from build123d import *

# Parameters (mm, degrees)
SKETCH_W        = 67.5
SKETCH_H        = 43.5
SKETCH_R        = 2
SKETCH_R_2      = 1.6
SKETCH_W_2      = 7.2
SKETCH_H_2      = 3.2
SKETCH_W_3      = 3.2
SKETCH_H_3      = 7.2
PAD_DEPTH       = 7
PAD001_DEPTH    = 5
SKETCH002_W     = 12
SKETCH002_H     = 12
PAD002_DEPTH    = 12
SKETCH003_R     = 4.2
POCKET_DEPTH    = 5
SKETCH004_R     = 1.7
POCKET001_DEPTH = 5
SKETCH005_R     = 1.7
POCKET002_DEPTH = 5


with BuildPart() as part:
    # Sketch → Pad (new body)
    with BuildSketch(Plane.XY):
        Rectangle(SKETCH_W, SKETCH_H)
        with Locations((0, -4.25)):
            Circle(SKETCH_R, mode=Mode.SUBTRACT)
        with Locations((-15.5, 11.25)):
            Circle(SKETCH_R_2, mode=Mode.SUBTRACT)
        with Locations((15.5, -19.75)):
            Circle(SKETCH_R_2, mode=Mode.SUBTRACT)
        with Locations((15.15, 18.15)):
            Rectangle(SKETCH_W_2, SKETCH_H_2, mode=Mode.SUBTRACT)
        with Locations((-25.15, 18.15)):
            Rectangle(SKETCH_W_2, SKETCH_H_2, mode=Mode.SUBTRACT)
        with Locations((30.15, 5.15)):
            Rectangle(SKETCH_W_3, SKETCH_H_3, mode=Mode.SUBTRACT)
        with Locations((30.15, -13.15)):
            Rectangle(SKETCH_W_3, SKETCH_H_3, mode=Mode.SUBTRACT)
    extrude(amount=PAD_DEPTH)

    # Sketch001 → Pad001 (new body)
    with BuildSketch(Plane.XY.offset(7)):
        Polygon((28.75, -21.75), (33.75, -21.75), (33.75, 21.75), (-33.75, 21.75), (-33.75, -21.75), (-21.75, -21.75), (-21.75, 16.75), (28.75, 16.75), align=None)
    extrude(amount=PAD001_DEPTH)

    # Sketch002 → Pad002 (new body)
    with BuildSketch(Plane.XY.offset(12)):
        with Locations((-27.75, -2)):
            Rectangle(SKETCH002_W, SKETCH002_H)
    extrude(amount=PAD002_DEPTH)

    # Sketch003 → Pocket (cut)
    with BuildSketch(Plane(origin=(-33.75, 0, 0), x_dir=(0, -1, 0), z_dir=(-1, 0, 0))):
        with Locations((2, 18)):
            Circle(SKETCH003_R)
    extrude(amount=-POCKET_DEPTH, mode=Mode.SUBTRACT)

    # Sketch004 → Pocket001 (cut)
    with BuildSketch(Plane(origin=(0, 21.75, 0), x_dir=(-1, 0, 0), z_dir=(0, 1, 0))):
        with Locations((25, 3.75)):
            Circle(SKETCH004_R)
        with Locations((-15, 3.75)):
            Circle(SKETCH004_R)
    extrude(amount=-POCKET001_DEPTH, mode=Mode.SUBTRACT)

    # Sketch005 → Pocket002 (cut)
    with BuildSketch(Plane.YZ.offset(33.75)):
        with Locations((5.15, 3.5)):
            Circle(SKETCH005_R)
        with Locations((-13.25, 3.5)):
            Circle(SKETCH005_R)
    extrude(amount=-POCKET002_DEPTH, mode=Mode.SUBTRACT)


solid = part.part
Model file for the job. Use its own axes, mm. A direction names the side the tool comes from. Coordinates: 2 decimals unless noted, no trailing zeros. Loops run counter-clockwise (first coordinate to the right, second up) from the corner with the lowest first, then second, coordinate; pieces in that order, holes last. Notation, with made-up numbers: (-39, 81.5) -> (3, 81.5) arc R11 cw to (3, 94.5) -> close; hole circle Ø6 at (-19.75, 16). An arc over 180 degrees is marked (long way). Use one line per item in the form item = value. Start each with the question number.
(1) Cut at D-D on z = 18. Give the cut face in (x, y), and give its area (3 significant figures).
(2) Tool access for faces 1 (the cylindrical face through (-31.285, -1.453, 22.164)), 2 (the flat face through (18.75, 18, 3)), 3 (the cylindrical face through (13.38, 20.76, 4.26)), 4 (the cylindrical face through (32.8, 6.7, 2.8)): list every direction of +Z, -Z, +X, -X, +Y, -Y with a clear straight run to the whole face (end or side of a thin tool).
(3) Probe probe 1 along X at (y, z) = (-16, 10); probe 2 along Z at (x, y) = (15, 20); probe 3 along Y at (x, z) = (12.5, 4.25). List the from-to ranges inside material, lowest first. Write a range as from..to.
(4) Cut at B-B on y = 11.25. Give the cut face in (x, z).
(5) Cut at C-C on y = -13.25. Give the cut face in (x, z).
(6) Pull direction Y, two halves, no side cores. Call faces 5 (the flat face through (0, 18, 12)), 6 (the flat face through (-28, 4, 18)), 7 (the flat face through (30, 1.55, 3)): pulls with the +Y half, pulls with the -Y half, needs draft (parallel to the pull), parting line crosses it, or undercut.
(7) Cut at A-A on x = 0. Give the cut face in (y, z).
(8) Flat gauge pins, fed straight in: pin 1 (1.5 mm diameter, centred on x = 6, z = 8.5, fed in from -Y); pin 2 (3 mm diameter, centred on x = -3.5, y = 4, fed in from +Z); pin 3 (1 mm diameter, centred on x = -25, y = 18.5, fed in from -Z). Where does each tip first touch, or does it go through?
Values:
q1.outline = (-33.75, -8) -> (-21.75, -8) -> (-21.75, 4) -> (-33.75, 4) -> (-33.75, 2.2) -> (-28.75, 2.2) -> (-28.75, -6.2) -> (-33.75, -6.2) -> close
q1.area = 102 mm2
q2.face_1 = -X
q2.face_2 = -Z
q2.face_3 = +Y
q2.face_4 = +X
q3.probe_1 = -33.75..-21.75, 28.75..33.75
q3.probe_2 = 0..2.05, 5.45..12
q3.probe_3 = -21.75..16.55, 19.75..21.75
q4.outline = (-33.75, 0) -> (-17.1, 0) -> (-17.1, 7) -> (-21.75, 7) -> (-21.75, 12) -> (-33.75, 12) -> close; (-13.9, 0) -> (33.75, 0) -> (33.75, 12) -> (28.75, 12) -> (28.75, 7) -> (-13.9, 7) -> close
q5.outline = (-33.75, 0) -> (28.55, 0) -> (28.55, 7) -> (-21.75, 7) -> (-21.75, 12) -> (-33.75, 12) -> close; (28.75, 7) -> (31.75, 7) -> (31.75, 5.2) -> (33.75, 5.2) -> (33.75, 12) -> (28.75, 12) -> close; (31.75, 0) -> (33.75, 0) -> (33.75, 1.8) -> (31.75, 1.8) -> close
q6.face_5 = needs draft
q6.face_6 = pulls with the +Y half
q6.face_7 = undercut
q7.outline = (-21.75, 0) -> (-6.25, 0) -> (-6.25, 7) -> (-21.75, 7) -> close; (-2.25, 0) -> (21.75, 0) -> (21.75, 12) -> (16.75, 12) -> (16.75, 7) -> (-2.25, 7) -> close
q8.pin_1 = 16.75
q8.pin_2 = 7
q8.pin_3 = 7
